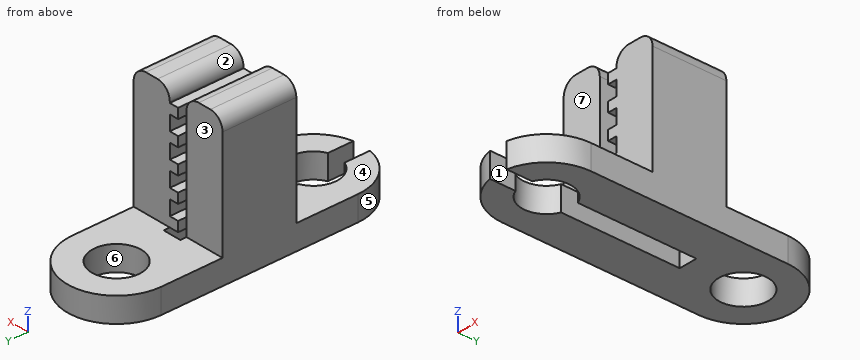
```python
from build123d import *

# Parameters (mm, degrees)
SKETCH_R            = 2
PAD_DEPTH           = 2
SKETCH001_W         = 6
SKETCH001_H         = 10
PAD001_DEPTH        = 4
SKETCH002_W         = 1.5
SKETCH002_H         = 15.5
POCKET_DEPTH        = 2
POCKET001_DEPTH     = 3.5
LINEARPATTERN_COUNT = 7
LINEARPATTERN_PITCH = 2
FILLET_R            = 1.1


with BuildPart() as part:
    # Sketch → Pad (new body)
    with BuildSketch(Plane.XY):
        with BuildLine():
            ThreePointArc((4, 8), (0, 12), (-4, 8))
            Line((-4, 8), (-4, -8))
            ThreePointArc((-4, -8), (0, -12), (4, -8))
            Line((4, 8), (4, -8))
        make_face()
        with Locations((0, 8)):
            Circle(SKETCH_R, mode=Mode.SUBTRACT)
        with Locations((0, -8)):
            Circle(SKETCH_R, mode=Mode.SUBTRACT)
    extrude(amount=PAD_DEPTH)

    # Sketch001 → Pad001 (join, symmetric)
    with BuildSketch(Plane.YZ):
        with Locations((0, 7)):
            Rectangle(SKETCH001_W, SKETCH001_H)
    extrude(amount=PAD001_DEPTH, both=True)

    # Sketch002 → Pocket (cut)
    with BuildSketch(Plane.XY):
        with Locations((0, -4.25)):
            Rectangle(SKETCH002_W, SKETCH002_H)
    extrude(amount=POCKET_DEPTH, mode=Mode.SUBTRACT)

    # Sketch003 → Pocket001 (cut, symmetric)
    with BuildSketch(Plane.XZ):
        Polygon((0, -1.2), (0, -2), (-0.75, -2), (-0.75, 0), (0.75, 0), (0.75, -1.2), align=None)
    pocket001 = extrude(amount=POCKET001_DEPTH, both=True, mode=Mode.SUBTRACT)

    # LinearPattern: Pocket001 ×7
    with Locations(*[(0, 0, i * LINEARPATTERN_PITCH) for i in range(1, LINEARPATTERN_COUNT)]):
        add(pocket001, mode=Mode.SUBTRACT)

    # Fillet
    fillet_edges = [part.edges().sort_by_distance(p)[0] for p in [
        (4, 0, 12),
        (0.75, 0, 12),
        (-0.75, 0, 12),
        (-4, 0, 12),
    ]]
    fillet(fillet_edges, radius=FILLET_R)


solid = part.part
```
Build history of the part. All positions in model axes, mm. Face numbers are marked on the shaded views. A direction names the side the tool comes from. Round coordinates to 2 decimals unless told otherwise and drop trailing zeros. Loops run counter-clockwise (first coordinate to the right, second up) from the corner with the lowest first, then second, coordinate; pieces in that order, holes last.
Item 1: Two-plate mould, pull along X, no slides. Class the marked faces 5, 6 and 7: released by +X, released by -X, zero draft, split by the parting line, or undercut.
Item 2: Saw through at D-D (y = 5.5). List the corners of the cut face in (x, z), then the cut area to 3 significant figures.
Item 3: Drill centre lines: line 1 along Y through (x, z) = (0, 1); line 2 along X through (y, z) = (-5, 1). Where is each one in solid material? Low to high.
Item 4: Saw through at B-B (z = 1.25). List the corners of the cut face in (x, y).
Item 5: Saw through at C-C (x = 3.5). List the corners of the cut face in (y, z), then the cut area to 3 significant figures.
Item 6: Saw through at A-A (z = 8.5). List the corners of the cut face in (x, y).
Item 7: Which spindle directions (+Z, -Z, +X, -X, +Y, -Y) get a long thin tool onto all of the face, cutting with end or side? Do the marked faces 1, 2, 3 and 4. Say none if no direction does.
Item 8: Pin check, flat tips, straight feed: P1, Ø4, axis at x = 0, z = 5, coming from the +Y side; P2, Ø2, axis at x = 1.5, z = 8.5, coming from the -Y side; P3, Ø3.5, axis at x = 0, y = 8, coming from the +Z side; P4, Ø1, axis at x = -2, y = -7.5, coming from the +Z side. Stop position of each tip, or through.
Worked answers:
1. face 5: released by -X
1. face 6: undercut
1. face 7: zero draft
2. outline: (-4, 0) - (4, 0) - (4, 2) - (-4, 2) - close
2. area: 16.0 mm2
3. line 1: y = 3.5 to 6, 10 to 12
3. line 2: x = -4 to -0.75, 0.75 to 4
4. outline: (-4, -8) arc R4 ccw to (-0.75, -11.93) - (-0.75, -9.85) arc R2 cw to (-0.75, -6.15) - (-0.75, 3.5) - (0.75, 3.5) - (0.75, -6.15) arc R2 cw to (0.75, -9.85) - (0.75, -11.93) arc R4 ccw to (4, -8) - (4, 8) arc R4 ccw to (-4, 8) - close; hole circle Ø4 at (0, 8)
5. outline: (-9.94, 0) - (9.94, 0) - (9.94, 2) - (3, 2) - (3, 11.82) - (-3, 11.82) - (-3, 2) - (-9.94, 2) - close
5. area: 98.7 mm2
6. outline: (-4, -3) - (-0.75, -3) - (-0.75, 3) - (-4, 3) - close; (0, -3) - (4, -3) - (4, 3) - (0, 3) - close
7. face 1: +Z, -Z, -Y
7. face 2: +Z, +Y, -Y
7. face 3: +Z, +X, -X, +Y
7. face 4: +Z, +X, -X, -Y
8. P1: stops at y = 3
8. P2: stops at y = -3
8. P3: passes through
8. P4: stops at z = 2
